```python
from build123d import *

# Parameters (mm, degrees)
F0_R     = 2.75
F0_W     = 9.4574374158
F0_H     = 1.2
F1_DEPTH = 14
F2_R     = 3.25
F3_DEPTH = 54
F4_DEPTH = 25
F5_SIZE  = 1.19999
F7_DEPTH = 7


# Not quite as in the source:
# - a fillet or chamfer is up to 0.001 mm smaller than in the source, because OpenCascade refuses the exact size


with BuildPart() as f1:
    # F0 (on Top) → F1 (new body)
    with BuildSketch(Plane.XY):
        with BuildLine():
            ThreePointArc((0, 3.95), (-2.7930717857, -2.7930717857), (3.95, 0))
            ThreePointArc((3.95, 0), (3.2094391954, 2.302607229), (1.2654430121, 3.7418115911))
            ThreePointArc((1.2654430121, 3.7418115911), (0.6412270328, 3.8976054049), (0, 3.95))
        make_face()
        Circle(F0_R, mode=Mode.SUBTRACT)
        with BuildLine():
            ThreePointArc((0, 3.95), (0.6412270328, 3.8976054049), (1.2654430121, 3.7418115911))
            Line((1.2654430121, 3.7418115911), (3.4641016151, 7.55))
            Line((3.4641016151, 7.55), (30.5358983849, 7.55))
            Line((30.5358983849, 7.55), (32.7345569879, 3.7418115911))
            ThreePointArc((32.7345569879, 3.7418115911), (33.3587729672, 3.8976054049), (34, 3.95))
            Line((34, 3.95), (31.2287187079, 8.75))
            Line((31.2287187079, 8.75), (21.7287187079, 8.75))
            Line((21.7287187079, 8.75), (12.2712812921, 8.75))
            Line((12.2712812921, 8.75), (2.7712812921, 8.75))
            Line((2.7712812921, 8.75), (0, 3.95))
        make_face()
        with Locations((17, 9.35)):
            Rectangle(F0_W, F0_H)
        with BuildLine():
            ThreePointArc((34, 3.95), (33.3587729672, 3.8976054049), (32.7345569879, 3.7418115911))
            ThreePointArc((32.7345569879, 3.7418115911), (31.697392771, -3.2094391954), (37.95, 0))
            ThreePointArc((37.95, 0), (36.7930717857, 2.7930717857), (34, 3.95))
        make_face()
        with Locations((34, 0)):
            Circle(F0_R, mode=Mode.SUBTRACT)
    extrude(amount=F1_DEPTH)

    # F2 (on face) → F3 (cut)
    with BuildSketch(Plane(origin=(0, 8.75, 0), x_dir=(-1, 0, 0), z_dir=(0, 1, 0))):
        with Locations((-17, 7)):
            Circle(F2_R)
    extrude(amount=-F3_DEPTH, mode=Mode.SUBTRACT)

    # F4 (cut): a face of the model
    f4_faces = [f1.faces().sort_by_distance(p)[0] for p in [
        (17, 8.75, 7),
    ]]
    extrude(f4_faces, amount=-F4_DEPTH, mode=Mode.SUBTRACT)

    # F5 (size 1.2 in the source; OpenCascade refuses exactly that, so slightly less here)
    f5_edges = [f1.edges().sort_by_distance(p)[0] for p in [
        (21.728719, 8.75, 7),
        (12.271281, 8.75, 7),
    ]]
    chamfer(f5_edges, length=F5_SIZE)

    # F6 (on face) → F7 (join)
    with BuildSketch(Plane.XZ.offset(-7.55)):
        Polygon((20.25, 0), (23.45, 0), (23.45, 12), (20.25, 12), (20.25, 7), align=None)
    extrude(amount=F7_DEPTH)


solid = f1.part
```
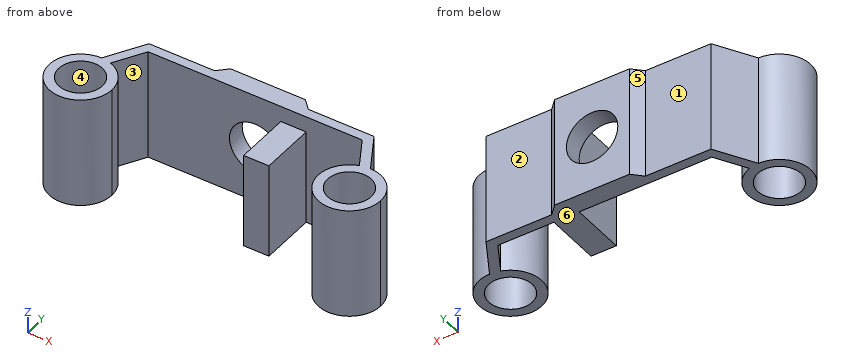
Model file for the job. Use its own axes, mm. Face numbers are marked on the shaded views. A direction names the side the tool comes from. Round coordinates to 2 decimals unless told otherwise and drop trailing zeros. Write each loop counter-clockwise with the first axis right and the second up, starting at its lowest first coordinate (ties: lowest second). Pieces come first, ordered by that corner, then holes. Notation, with made-up numbers: (2.25, -1) - (60.25, -1) arc R20 cw to (60.25, 34) - close; hole circle Ø9 at (30, 4). An arc over 180 degrees is marked (long way). Use CSV: the item, a comma, the result in double quotes. Start each with the question number.
Item 1: Band-saw the part on A-A (z = 7.75). State how many separate pieces and enclosed holes the cut face has, and give its area (3 significant figures).
Item 2: Tool access for the marked faces 1, 2 and 3: list every direction of +Z, -Z, +X, -X, +Y, -Y with a clear straight run to the whole face (end or side of a thin tool).
Item 3: Band-saw the part on D-D (y = 9.25). Write the cut outline in (x, z), and give its area (3 significant figures).
Item 4: Band-saw the part on B-B (x = 15). Write the cut outline in (y, z).
Item 5: Two-plate mould, pull along X, no slides. Class the marked faces 4, 5 and 6: released by +X, released by -X, zero draft, split by the parting line, or undercut.
Item 6: Pin check, flat tips, straight feed: P1, Ø3, axis at x = 0.5, z = 4, coming from the -Y side; P2, Ø1, axis at y = 6, z = 2.5, coming from the -X side; P3, Ø2, axis at y = 5, z = 5, coming from the +X side; P4, Ø2.5, axis at x = 26.5, z = 5, coming from the +Y side. Stop position of each tip, or through.
Item 7: Drill centre lines: L1, parallel to Z at x = 17, y = 8.25; L2, parallel to X at y = -2, z = 5; L3, parallel to X at y = 3, z = 10. Where is each one in solid material? Low to high. Write a range as [from, to].
Checked values:
1,separate pieces,"2"
1,enclosed holes,"2"
1,area,"116 mm²"
2,face 1,"+Z, -Z, -X, +Y"
2,face 2,"+Z, -Z, +X, +Y"
2,face 3,"+Z, -Z"
3,outline,"(11.57, 0) - (22.43, 0) - (22.43, 14) - (11.57, 14) - close; hole circle Ø6.5 at (17, 7)"
3,area,"119 mm²"
4,outline,"(7.55, 0) - (9.95, 0) - (9.95, 4.44) - (7.55, 4.44) - close; (7.55, 9.56) - (9.95, 9.56) - (9.95, 14) - (7.55, 14) - close"
5,face 4,"undercut"
5,face 5,"released by -X"
5,face 6,"zero draft"
6,P1,"stops at y = -3.95"
6,P2,"stops at x = 0.89"
6,P3,"stops at x = 33.97"
6,P4,"stops at y = 8.75"
7,L1,"z = [0, 3.75], [10.25, 14]"
7,L2,"x = [-3.41, -1.89], [1.89, 3.41], [30.59, 32.11], [35.89, 37.41]"
7,L3,"x = [-2.57, 2.57], [20.25, 23.45], [31.43, 36.57]"
